Part model, mm, in its own coordinate system. A direction names the side the tool comes from. Coordinates: 2 decimals unless noted, no trailing zeros. Write each loop counter-clockwise with the first axis right and the second up, starting at its lowest first coordinate (ties: lowest second). Pieces come first, ordered by that corner, then holes. Notation, with made-up numbers: (64, 42) - (83, 42) arc R11 ccw to (83, 47) - close; hole circle Ø9 at (-21.5, 57.25). An arc over 180 degrees is marked (long way). Use one line per item in the form item = value. Start each with the question number.
from build123d import *

# Parameters (mm, degrees)
SKETCH1_R           = 2.0828
BOSS_EXTRUDE1_DEPTH = 6.35
BOSS_EXTRUDE2_DEPTH = 12.7
SKETCH3_W           = 10.16
SKETCH3_H           = 8.980256121
SKETCH3_R           = 2.0828
CUT_EXTRUDE2_DEPTH  = 81.532421421
CUT_EXTRUDE3_DEPTH  = 2.54


with BuildPart() as part:
    # Sketch1 → Boss-Extrude1 (new body)
    with BuildSketch(Plane(origin=(0, 0, 0), x_dir=(0, 0, -1), z_dir=(1, 0, 0))):
        with BuildLine():
            Line((-25.4, 31.75), (25.4, 31.75))
            ThreePointArc((25.4, 31.75), (27.830039796, 31.266635031), (29.890128061, 29.890128061))
            Line((29.890128061, 29.890128061), (43.860128061, 15.920128061))
            ThreePointArc((43.860128061, 15.920128061), (45.236635031, 13.860039796), (45.72, 11.43))
            Line((45.72, 11.43), (45.72, -11.43))
            ThreePointArc((45.72, -11.43), (45.236635031, -13.860039796), (43.860128061, -15.920128061))
            Line((43.860128061, -15.920128061), (29.890128061, -29.890128061))
            ThreePointArc((29.890128061, -29.890128061), (27.830039796, -31.266635031), (25.4, -31.75))
            Line((25.4, -31.75), (-25.4, -31.75))
            ThreePointArc((-25.4, -31.75), (-27.830039796, -31.266635031), (-29.890128061, -29.890128061))
            Line((-29.890128061, -29.890128061), (-43.860128061, -15.920128061))
            ThreePointArc((-43.860128061, -15.920128061), (-45.236635031, -13.860039796), (-45.72, -11.43))
            Line((-45.72, -11.43), (-45.72, 11.43))
            ThreePointArc((-45.72, 11.43), (-45.236635031, 13.860039796), (-43.860128061, 15.920128061))
            Line((-43.860128061, 15.920128061), (-29.890128061, 29.890128061))
            ThreePointArc((-29.890128061, 29.890128061), (-27.830039796, 31.266635031), (-25.4, 31.75))
        make_face()
        with Locations((38.1, 12.7)):
            Circle(SKETCH1_R, mode=Mode.SUBTRACT)
        with Locations(Location((38.1, -12.7, 0), (0, 0, 180))):
            Circle(SKETCH1_R, mode=Mode.SUBTRACT)
        with Locations((-38.1, -12.7)):
            Circle(SKETCH1_R, mode=Mode.SUBTRACT)
        with Locations(Location((-38.1, 12.7, 0), (0, 0, 180))):
            Circle(SKETCH1_R, mode=Mode.SUBTRACT)
        with BuildLine():
            Line((-19.05, 25.4), (19.05, 25.4))
            ThreePointArc((19.05, 25.4), (23.540128061, 23.540128061), (25.4, 19.05))
            Line((25.4, 19.05), (25.4, -19.05))
            ThreePointArc((25.4, -19.05), (23.540128061, -23.540128061), (19.05, -25.4))
            Line((19.05, -25.4), (-19.05, -25.4))
            ThreePointArc((-19.05, -25.4), (-23.540128061, -23.540128061), (-25.4, -19.05))
            Line((-25.4, -19.05), (-25.4, 19.05))
            ThreePointArc((-25.4, 19.05), (-23.540128061, 23.540128061), (-19.05, 25.4))
        make_face(mode=Mode.SUBTRACT)
    extrude(amount=BOSS_EXTRUDE1_DEPTH)

    # Sketch2 → Boss-Extrude2 (add)
    with BuildSketch(Plane(origin=(6.35, 0, 0), x_dir=(0, 0, -1), z_dir=(1, 0, 0))):
        with BuildLine():
            Line((25.4, 31.75), (-25.4, 31.75))
            ThreePointArc((-25.4, 31.75), (-27.830039796, 31.266635031), (-29.890128061, 29.890128061))
            Line((-29.890128061, 29.890128061), (-34.380256121, 25.4))
            Line((-34.380256121, 25.4), (-19.05, 25.4))
            Line((-19.05, 25.4), (19.05, 25.4))
            Line((19.05, 25.4), (34.380256121, 25.4))
            Line((34.380256121, 25.4), (29.890128061, 29.890128061))
            ThreePointArc((29.890128061, 29.890128061), (27.830039796, 31.266635031), (25.4, 31.75))
        make_face()
    boss_extrude2 = extrude(amount=BOSS_EXTRUDE2_DEPTH)

    # Mirror1: Boss-Extrude2 across plane
    add(boss_extrude2.mirror(Plane.ZX))

    # Sketch3 → Cut-Extrude2 (cut, through all)
    with BuildSketch(Plane.XZ.offset(31.75)):
        with Locations((13.97, 29.890128061)):
            Rectangle(SKETCH3_W, SKETCH3_H)
        Polygon((8.89, 22.86), (19.05, 12.7), (19.05, 25.4), (8.89, 25.4), align=None)
        with Locations((13.97, -29.890128061)):
            Rectangle(SKETCH3_W, SKETCH3_H)
        Polygon((8.89, -25.4), (19.05, -25.4), (19.05, -12.7), (8.89, -22.86), align=None)
        with Locations(Location((13.97, 0, 0), (0, 0, 270))):
            Circle(SKETCH3_R)
    extrude(amount=-CUT_EXTRUDE2_DEPTH, mode=Mode.SUBTRACT)

    # Sketch5 → Cut-Extrude3 (cut)
    with BuildSketch(Plane(origin=(6.35, 0, 0), x_dir=(0, 0, -1), z_dir=(1, 0, 0))):
        with BuildLine():
            Line((-36.83, 19.05), (-45.72, 19.05))
            Line((-45.72, 19.05), (-45.72, -19.05))
            Line((-45.72, -19.05), (-36.83, -19.05))
            ThreePointArc((-36.83, -19.05), (-32.339871939, -17.190128061), (-30.48, -12.7))
            Line((-30.48, -12.7), (-30.48, 12.7))
            ThreePointArc((-30.48, 12.7), (-32.339871939, 17.190128061), (-36.83, 19.05))
        make_face()
    extrude(amount=-CUT_EXTRUDE3_DEPTH, mode=Mode.SUBTRACT)


solid = part.part
Q1. Slice it at D-D (x = 5). List the corners of the cut face in (y, z).
Q2. Drill centre lines: probe 1 along Y at (x, z) = (2.2, 38.1); probe 2 along Y at (x, z) = (7.5, -18); probe 3 along X at (y, z) = (-27, 0). Where is each one in solid material? Low to high.
Q3. Slice it at C-C (x = 10). List the corners of the cut face in (y, z).
Q4. Pin check, flat tips, straight feed: P1, Ø1.9, axis at y = -30, z = -29, coming from the +X side; P2, Ø8, axis at y = 15, z = -26.5, coming from the +X side; P3, Ø3.5, axis at x = 13.97, z = 0, coming from the -Y side; P4, Ø3, axis at x = 5.5, z = 38.5, coming from the -Y side. Stop position of each tip, or through.
Q5. Slice it at B-B (z = 4.5). List the corners of the cut face in (x, y).
Q6. Mould opens along Z. For faces 1 (the cylindrical face through (1.88, -12.61, 40.18)), 2 (the cylindrical face through (1.878, 12.074, 40.087)), 3 (the cylindrical face through (5.1, 17.14, 32.29)), 4 (the flat face through (7, -31.75, 0)) say: released by +Z, released by -Z, zero draft, split by the parting line, or undercut.
Q7. Which spindle directions (+Z, -Z, +X, -X, +Y, -Y) get a long thin tool onto all of the face, cutting with end or side? Do faces 5 (the cylindrical face through (3.13, -23.59, 23.49)), 6 (the flat face through (8.89, 28, 27)), 7 (the flat face through (8.89, -28, -27)), 8 (the flat face through (19.05, -29, 0)), 9 (the cylindrical face through (12.12, 28.53, -0.96)). Say none if no direction does.
Q8. Slice it at A-A (y = 2.5). List the corners of the cut face in (x, z).
Solution:
q1.outline = (-31.75, -25.4) arc R6.35 ccw to (-29.89, -29.89) - (-15.92, -43.86) arc R6.35 ccw to (-11.43, -45.72) - (11.43, -45.72) arc R6.35 ccw to (15.92, -43.86) - (29.89, -29.89) arc R6.35 ccw to (31.75, -25.4) - (31.75, 25.4) arc R6.35 ccw to (29.89, 29.89) - (19.05, 40.73) - (19.05, 36.83) arc R6.35 cw to (12.7, 30.48) - (-12.7, 30.48) arc R6.35 cw to (-19.05, 36.83) - (-19.05, 40.73) - (-29.89, 29.89) arc R6.35 ccw to (-31.75, 25.4) - close; hole (-25.4, -19.05) arc R6.35 ccw to (-19.05, -25.4) - (19.05, -25.4) arc R6.35 ccw to (25.4, -19.05) - (25.4, 19.05) arc R6.35 ccw to (19.05, 25.4) - (-19.05, 25.4) arc R6.35 ccw to (-25.4, 19.05) - close; hole circle Ø4.17 at (-12.7, -38.1); hole circle Ø4.17 at (12.7, -38.1)
q2.probe_1 = -21.68 to -14.78, -10.62 to 10.62, 14.78 to 21.68
q2.probe_2 = -31.75 to -25.4, 25.4 to 31.75
q2.probe_3 = 0 to 11.89, 16.05 to 19.05
q3.outline = (-31.75, -21.75) - (-25.4, -21.75) - (-25.4, 21.75) - (-31.75, 21.75) - close; (25.4, -21.75) - (31.75, -21.75) - (31.75, 21.75) - (25.4, 21.75) - close
q4.P1 = 8.89
q4.P2 = 6.35
q4.P3 = through
q4.P4 = -22.78
q5.outline = (0, -31.75) - (19.05, -31.75) - (19.05, -25.4) - (0, -25.4) - close; (0, 25.4) - (19.05, 25.4) - (19.05, 31.75) - (0, 31.75) - close
q6.face_1 = undercut
q6.face_2 = undercut
q6.face_3 = released by +Z
q6.face_4 = zero draft
q7.face_5 = +X, -X
q7.face_6 = +Z, +X, +Y, -Y
q7.face_7 = -Z, +X, +Y, -Y
q7.face_8 = +Z, -Z, +X, +Y, -Y
q7.face_9 = +Y, -Y
q8.outline = (0, -45.72) - (6.35, -45.72) - (6.35, -25.4) - (0, -25.4) - close; (0, 25.4) - (6.35, 25.4) - (6.35, 30.48) - (3.81, 30.48) - (3.81, 45.72) - (0, 45.72) - close
